Here's how the part is built. I have some questions about the finished solid (model axes, mm). Coordinates: 2 decimals unless noted, no trailing zeros. Loops run counter-clockwise (first coordinate to the right, second up) from the corner with the lowest first, then second, coordinate; pieces in that order, holes last.
Autodesk Inventor part; units mm, degrees
ref_plane "YZ Plane" through (0, 0, 0) normal (1, 0, 0) x (0, 1, 0)
ref_plane "XZ Plane" through (0, 0, 0) normal (0, 1, 0) x (-1, 0, 0)
ref_plane "XY Plane" through (0, 0, 0) normal (0, 0, 1) x (1, 0, 0)
sketch "Boceto1" plane through (0, 0, 0) normal (0, 0, 1) x (1, 0, 0)
  line L0 (-250, -215) -> (250, -215)
  line L1 (250, -215) -> (250, 215)
  line L2 (250, 215) -> (-250, 215)
  line L3 (-250, 215) -> (-250, -215)
  line L4 (-250, -215) -> (250, 215) construction
  line L5 (250, -215) -> (-250, 215) construction
  point P0 (0, 0)
  dimension "d0" = 500
  dimension "d1" = 430
extrude "Extrusión1" add sketch "Boceto1" along normal blind 20
sketch "Boceto7" plane through (0, 0, 20) normal (0, 0, 1) x (1, 0, 0)
  line L0 (-135.0434, 135.4344) -> (-155.0434, 135.4344)
  line L1 (-155.0434, 170.4344) -> (-155.0434, 100.4344)
  line L2 (-145.0434, 135.4344) -> (-145.0434, 185.4344)
  line L3 (-70.0434, 185.4344) -> (-200.0434, 185.4344)
  line L4 (-145.0434, 170.4344) -> (-145.0434, 185.4344)
  line L5 (-145.0434, 185.4344) -> (-145.0434, 177.9344)
  line L6 (-145.0434, 135.4344) -> (-70.0434, 135.4344)
  line L7 (-70.0434, 85.4344) -> (-70.0434, 185.4344)
  line L8 (-95.0434, 170.4344) -> (-95.0434, 100.4344)
  line L9 (-95.0434, 135.4344) -> (-70.0434, 135.4344)
  line L10 (-82.5434, 135.4344) -> (-82.5434, 155.4344)
  circle A0 centre (-145.0434, 177.9344) radius 3
  circle A1 centre (-82.5434, 155.4344) radius 3
  circle A2 centre (-145.0434, 92.9344) radius 3
  circle A3 centre (-82.5434, 115.4344) radius 3
  line L11 (-250, 215) -> (-250, -215)
  line L12 (-250, 215) -> (-200, 215)
  line L13 (-200, 215) -> (-200, 185)
  line L14 (-250, 0) -> (0, 0)
  line L15 (250, -215) -> (-250, -215)
  line L16 (135.0434, -135.4344) -> (155.0434, -135.4344)
  line L17 (155.0434, -170.4344) -> (155.0434, -100.4344)
  line L18 (145.0434, -135.4344) -> (70.0434, -135.4344)
  line L19 (-250, -215) -> (250, -215)
  line L20 (70.0434, -185.4344) -> (200.0434, -185.4344)
  line L21 (145.0434, -185.4344) -> (145.0434, -177.9344)
  line L22 (145.0434, -170.4344) -> (145.0434, -185.4344)
  circle A4 centre (145.0434, -177.9344) radius 3
  circle A5 centre (145.0434, -92.9344) radius 3
  line L23 (200, -215) -> (200, -185)
  line L24 (145.0434, -135.4344) -> (145.0434, -185.4344)
  line L25 (250, -215) -> (200, -215)
  line L26 (95.0434, -170.4344) -> (95.0434, -100.4344)
  line L27 (70.0434, -85.4344) -> (70.0434, -185.4344)
  circle A6 centre (82.5434, -115.4344) radius 3
  line L28 (82.5434, -135.4344) -> (82.5434, -155.4344)
  circle A7 centre (82.5434, -155.4344) radius 3
  line L29 (95.0434, -135.4344) -> (70.0434, -135.4344)
  point P0 (250, 215)
  dimension "d22" = 20
  dimension "d23" = 6
  dimension "d24" = 6
  dimension "d25" = 50
  dimension "d26" = 30
extrude "Extrusión7" add sketch "Boceto7" along normal blind 50 contours A1 | A0 L2 | L2 A0 | A2 | A3
extrude "Extrusión8" add sketch "Boceto7" along normal blind 50 contours A7 | A4 L22 L21 | L21 L22 A4 | A5 | A6
properties part number "Placa"
Q1. Suppose I cut it at B-B on x = -102.5. Write out the boundary of the cut face in (y, z), and give its area (3 significant figures).
Q2. Suppose I cut it at C-C on y = 142. Write out the boundary of the cut face in (x, z).
Q3. Will this pin go through, and if not, where does the flat tip stop? P1, Ø1, axis at y = 113, z = 51.5, coming from the +X side.
Q4. We'd pull the mould along Z, two halves only. Please class faces 1 (the flat face through (250, -3, 10)), 2 (the flat face through (-3, 3, 20)), 3 (the flat face through (-3, 3, 0)): pulls with the +Z half, pulls with the -Z half, needs draft (parallel to the pull), parting line crosses it, or undercut.
Q5. Please list where this line runs through material, in increasing order: probe 1 along Z at (x, y) = (-126, -164.5).
Q6. Suppose I cut it at A-A on z = 26.5. Write out the boundary of the cut face in (x, y).
Check values:
1. outline: (-215, 0) - (215, 0) - (215, 20) - (-215, 20) - close
1. area: 8,600 mm2
2. outline: (-250, 0) - (250, 0) - (250, 20) - (-250, 20) - close
3. P1: stops at x = -80.25
4. face 1: needs draft
4. face 2: pulls with the +Z half
4. face 3: pulls with the -Z half
5. probe 1: z = 0 to 20
6. outline: circle Ø6 at (-145.04, 92.93); circle Ø6 at (-145.04, 177.93); circle Ø6 at (-82.54, 115.43); circle Ø6 at (-82.54, 155.43); circle Ø6 at (82.54, -155.43); circle Ø6 at (82.54, -115.43); circle Ø6 at (145.04, -177.93); circle Ø6 at (145.04, -92.93)
